Here's the drawing with two shaded views (mm, measured from the low corner). I have some questions. A direction names the side the tool comes from. Round coordinates to 2 decimals unless told otherwise and drop trailing zeros. Order: outer loops, then holes, each group sorted by start corner. A loop starts at its lowest first (then second) coordinate and runs counter-clockwise, first axis right, second up. Notation, with made-up numbers: (-26.75, -38.75) -> (-16.75, -38.75) arc R24 ccw to (-16.75, -15.75) -> close; hole circle Ø11 at (-35.75, 12). An arc over 180 degrees is marked (long way). Answer in a Markdown table with one row per item.
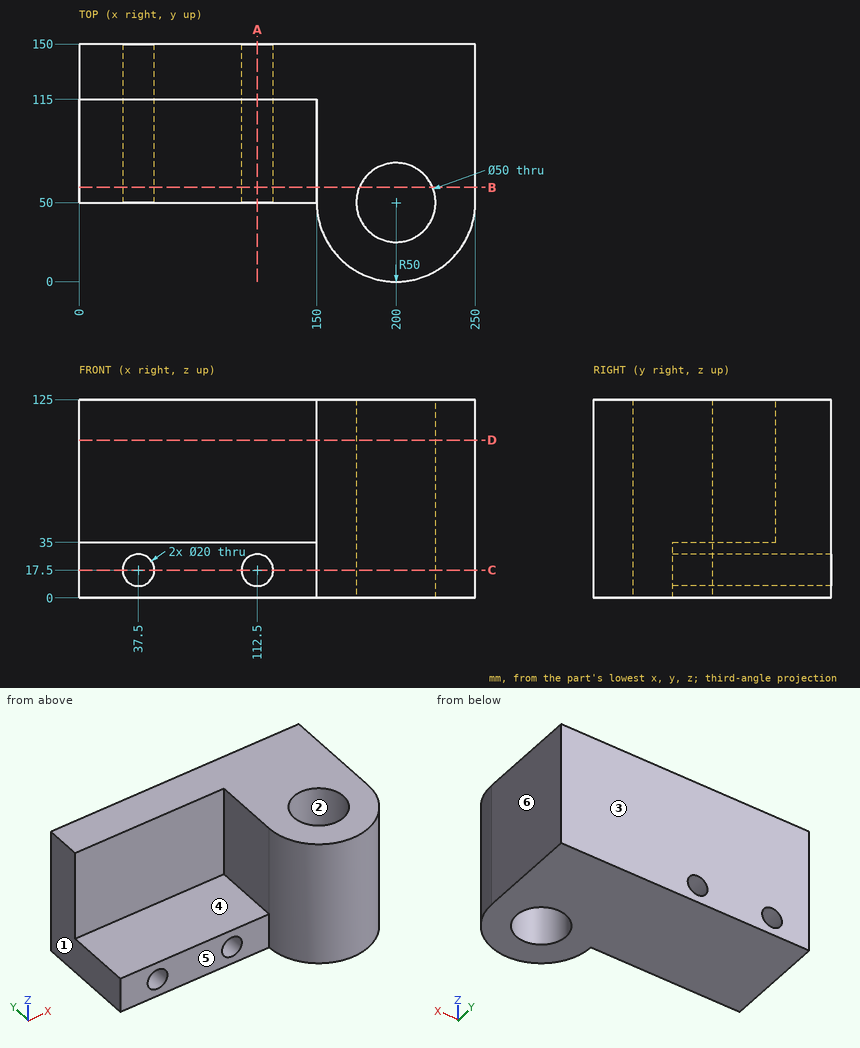
1. Suppose I cut it at B-B on y = 59.5. Write out the boundary of the cut face in (x, z), then the cut area to 3 significant figures.
Numbers:
| item | result |
|---|---|
| outline | (0, 0) -> (176.88, 0) -> (176.88, 125) -> (150, 125) -> (150, 35) -> (0, 35) -> close; (223.12, 0) -> (250, 0) -> (250, 125) -> (223.12, 125) -> close; hole circle Ø20 at (37.5, 17.5); hole circle Ø20 at (112.5, 17.5) |
| area | 11,300 mm2 |
2. We'd pull the mould along X, two halves only. Please class the marked faces 1, 2 and 3: released by +X, released by -X, zero draft, split by the parting line, or undercut.
Numbers:
| item | result |
|---|---|
| face 1 | released by -X |
| face 2 | undercut |
| face 3 | zero draft |
3. Suppose I cut it at C-C on z = 17.5. Write out the boundary of the cut face in (x, y), then the cut area to 3 significant figures.
Numbers:
| item | result |
|---|---|
| outline | (0, 50) -> (27.5, 50) -> (27.5, 150) -> (0, 150) -> close; (47.5, 50) -> (102.5, 50) -> (102.5, 150) -> (47.5, 150) -> close; (122.5, 50) -> (150, 50) arc R50 ccw to (250, 50) -> (250, 150) -> (122.5, 150) -> close; hole circle Ø50 at (200, 50) |
| area | 23,000 mm2 |
4. For the marked faces 4, 5 and 6, which set-ups out of +Z, -Z, +X, -X, +Y, -Y let a thin tool reach every point of the face, with its end or its side?
Numbers:
| item | result |
|---|---|
| face 4 | +Z, -X, -Y |
| face 5 | +Z, -Z, -X, -Y |
| face 6 | +Z, -Z, +X, +Y, -Y |
5. Please list where these lines run through material, in increasing order: line 1 along X through (y, z) = (104, 17); line 2 along Y through (x, z) = (199, 78); line 3 along X through (y, z) = (99.5, 15).
Numbers:
| item | result |
|---|---|
| line 1 | x = 0 to 27.51, 47.49 to 102.51, 122.49 to 250 |
| line 2 | y = 0.01 to 25.02, 74.98 to 150 |
| line 3 | x = 0 to 27.82, 47.18 to 102.82, 122.18 to 250 |
6. Suppose I cut it at D-D on z = 99.5. Write out the boundary of the cut face in (x, y), then the cut area to 3 significant figures.
Numbers:
| item | result |
|---|---|
| outline | (0, 115) -> (150, 115) -> (150, 50) arc R50 ccw to (250, 50) -> (250, 150) -> (0, 150) -> close; hole circle Ø50 at (200, 50) |
| area | 17,200 mm2 |
7. For pin 1 Ø16 at (x, z) = (37.5, 17.5) entering from +Y; pin 2 Ø10 at (x, z) = (124, 65.5) entering from -Y; pin 3 Ø19.5 at (x, y) = (100, 71) entering from +Z, each with a flat end and sliding along its axis, tell me the tip position at first contact or that it passes through.
Numbers:
| item | result |
|---|---|
| pin 1 | passes through |
| pin 2 | stops at y = 115 |
| pin 3 | stops at z = 35 |
8. Suppose I cut it at A-A on x = 112.5. Write out the boundary of the cut face in (y, z).
Numbers:
| item | result |
|---|---|
| outline | (50, 0) -> (150, 0) -> (150, 7.5) -> (50, 7.5) -> close; (50, 27.5) -> (150, 27.5) -> (150, 125) -> (115, 125) -> (115, 35) -> (50, 35) -> close |
